```python
from build123d import *

# Parameters (mm, degrees)
SALIENTE_EXTRUIR1_DEPTH = 10
CROQUIS2_R              = 6.418605164
SALIENTE_EXTRUIR2_DEPTH = 5


with BuildPart() as part:
    # Croquis1 → Saliente-Extruir1 (new body)
    with BuildSketch(Plane.XY):
        with BuildLine():
            Line((-55.369792261, 7.493056697), (-40.369792261, 7.493056697))
            ThreePointArc((-40.369792261, 7.493056697), (-30.369792261, -2.506943303), (-40.369792261, -12.506943303))
            Line((-40.369792261, -12.506943303), (-55.369792261, -12.506943303))
            ThreePointArc((-55.369792261, -12.506943303), (-65.369792261, -2.506943303), (-55.369792261, 7.493056697))
        make_face()
    extrude(amount=SALIENTE_EXTRUIR1_DEPTH)

    # Croquis2 → Saliente-Extruir2 (add)
    with BuildSketch(Plane.XY.offset(10)):
        with Locations((-46.174536974, -2.897909692)):
            Circle(CROQUIS2_R)
    extrude(amount=SALIENTE_EXTRUIR2_DEPTH)


solid = part.part
```
Here's how the part is built. I have some questions about the finished solid (model axes, mm). A direction names the side the tool comes from. Coordinates: 2 decimals unless noted, no trailing zeros. Loops run counter-clockwise (first coordinate to the right, second up) from the corner with the lowest first, then second, coordinate; pieces in that order, holes last. Notation, with made-up numbers: (-26.5, 41) - (-21.5, 41) arc R33 ccw to (-21.5, 73) - close; hole circle Ø2 at (-39.75, 26.5). An arc over 180 degrees is marked (long way). Return JSON: item names as keys, results as strings. Group by question number.
Item 1: If we section it at C-C on z = 7.5: Write out the boundary of the cut face in (x, y).
Item 2: If we section it at B-B on x = -53.5: Write out the boundary of the cut face in (y, z), and give its area (3 significant figures).
Item 3: If we section it at D-D on x = -49: Write out the boundary of the cut face in (y, z), and give its area (3 significant figures).
Item 4: If we section it at A-A on y = -3.5: Write out the boundary of the cut face in (x, z), and give its area (3 significant figures).
Item 5: Will these pins go through, and if not, where does the flat tip stop? P1, Ø8, axis at x = -57, y = -0.5, coming from the +Z side; P2, Ø5, axis at x = -50.5, z = 13, coming from the -Y side; P3, Ø1, axis at y = -7.5, z = 5, coming from the +X side.
Item 6: On a 3-axis mill with a long thin cutter (end or side, diameter ignored), from which of +Z, -Z, +X, -X, +Y, -Y can I reach the whole of each face in a straight line? I mean faces 1 (the face through (-52, -7, 10)), 2 (the face through (-30.372, -2.287, 4.93)). Say none if no direction works.
Item 7: I need wall thicknesses on line 1 (Z direction, x = -46.5, y = 4.25); line 2 (Y direction, x = -46.5, z = 14.5); line 3 (Y direction, x = -40, z = 6.75). Which ranges of each line are inside material? Lowest first, please. Write a range as from..to.
Calculated:
{
 "1": {"outline": "(-55.37, -12.51) - (-40.37, -12.51) arc R10 ccw to (-40.37, 7.49) - (-55.37, 7.49) arc R10 ccw to start"},
 "2": {"outline": "(-12.51, 0) - (7.49, 0) - (7.49, 10) - (-12.51, 10) - close", "area": "200 mm^2"},
 "3": {"outline": "(-12.51, 0) - (7.49, 0) - (7.49, 10) - (2.87, 10) - (2.87, 15) - (-8.66, 15) - (-8.66, 10) - (-12.51, 10) - close", "area": "258 mm^2"},
 "4": {"outline": "(-65.32, 0) - (-30.42, 0) - (-30.42, 10) - (-39.78, 10) - (-39.78, 15) - (-52.56, 15) - (-52.56, 10) - (-65.32, 10) - close", "area": "413 mm^2"},
 "5": {"P1": "stops at z = 10", "P2": "stops at y = -9.05", "P3": "stops at x = -31.44"},
 "6": {"face 1": "+Z", "face 2": "+Z, -Z, +X"},
 "7": {"line 1": "z = 0..10", "line 2": "y = -9.31..3.51", "line 3": "y = -12.5..7.49"}
}
